Geometry check sheet. Reference: the model listing, model coordinates, mm. Face numbers are marked on the shaded views. Round coordinates to 2 decimals unless told otherwise and drop trailing zeros. Loops run counter-clockwise (first coordinate to the right, second up) from the corner with the lowest first, then second, coordinate; pieces in that order, holes last.
```python
from build123d import *

# Parameters (mm, degrees)
SKETCH1_R           = 38.5
SKETCH1_R_2         = 36.5
BOSS_EXTRUDE1_DEPTH = 257
SKETCH3_W           = 21
SKETCH3_H           = 31
CUT_EXTRUDE1_DEPTH  = 50
SKETCH8_W           = 16.314187307
SKETCH8_H           = 32.341181037
CUT_EXTRUDE4_DEPTH  = 40


with BuildPart() as part:
    # Sketch1 → Boss-Extrude1 (new body)
    with BuildSketch(Plane(origin=(0, 0, 0), x_dir=(1, 0, 0), z_dir=(0, 1, 0))):
        with Locations(Location((0, 0, 0), (0, 0, 270))):
            Circle(SKETCH1_R)
        with Locations(Location((0, 0, 0), (0, 0, 270))):
            Circle(SKETCH1_R_2, mode=Mode.SUBTRACT)
    extrude(amount=BOSS_EXTRUDE1_DEPTH)

    # Sketch3 → Cut-Extrude1 (cut)
    with BuildSketch(Plane(origin=(0, 0, 0), x_dir=(0, 0, -1), z_dir=(1, 0, 0))):
        with Locations((-19.608340935, 67.295682387)):
            Rectangle(SKETCH3_W, SKETCH3_H)
    extrude(amount=-CUT_EXTRUDE1_DEPTH, mode=Mode.SUBTRACT)

    # Sketch8 → Cut-Extrude4 (cut)
    with BuildSketch(Plane.XY):
        with Locations((22.858818879, 14.180131948)):
            Rectangle(SKETCH8_W, SKETCH8_H)
    extrude(amount=CUT_EXTRUDE4_DEPTH, mode=Mode.SUBTRACT)


solid = part.part
```
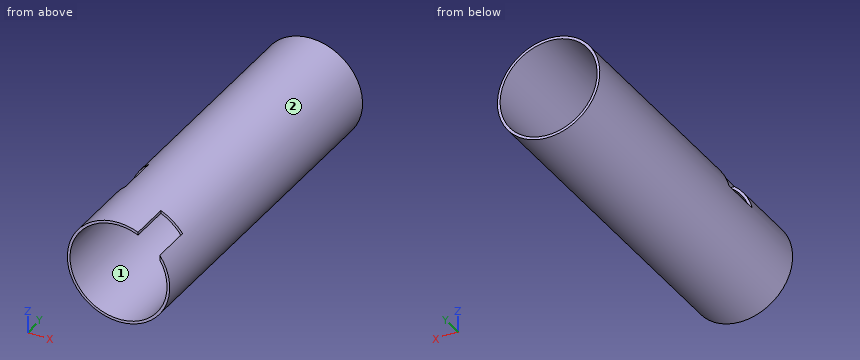
1) Sectioned sample at C-C, the plane x = -31.5. Record the cut outline in (y, z).
Report:
outline: (0, -22.14) - (257, -22.14) - (257, -18.44) - (0, -18.44) - close; (0, 18.44) - (51.8, 18.44) - (51.8, 22.14) - (0, 22.14) - close; (82.8, 18.44) - (257, 18.44) - (257, 22.14) - (82.8, 22.14) - close
2) Sectioned sample at D-D, the plane y = 91.5. Record the cut outline in (x, z).
Report:
outline: circle Ø77 at (0, 0); hole circle Ø73 at (0, 0)
3) Scan lines: line 1 along Z through (x, y) = (-1.5, 112.5); line 2 along X through (y, z) = (114, 0); line 3 along X through (y, z) = (20, 19). Record each from-to range of solid material in increasing order.
Report:
line 1: z = -38.47 to -36.47, 36.47 to 38.47
line 2: x = -38.5 to -36.5, 36.5 to 38.5
line 3: x = -33.49 to -31.16, 31.16 to 33.49
4) Sectioned sample at A-A, the plane x = 0. Record the cut outline in (y, z), then the cut area to 3 significant figures.
Report:
outline: (0, -38.5) - (257, -38.5) - (257, -36.5) - (0, -36.5) - close; (0, 36.5) - (257, 36.5) - (257, 38.5) - (0, 38.5) - close
area: 1,030 mm2
5) Gauge pin test, flat ends, axial feed: pin 1 (6 mm diameter, centred on y = 83, z = 29.5, fed in from -X); pin 2 (12 mm diameter, centred on x = -25, y = 174, fed in from -Z); pin 3 (3 mm diameter, centred on y = 97, z = 13.5, fed in from +X); pin 4 (5 mm diameter, centred on x = -29.5, z = 20.5, fed in from +Y). Record the tip position at first contact, or that the pin passes through.
Report:
pin 1: stops at x = -27.93
pin 2: stops at z = -33.49
pin 3: stops at x = 36.58
pin 4: stops at y = 257
6) Sectioned sample at B-B, the plane z = 0. Record the cut outline in (x, y), then the cut area to 3 significant figures.
Report:
outline: (-38.5, 0) - (-36.5, 0) - (-36.5, 257) - (-38.5, 257) - close; (36.5, 0) - (38.5, 0) - (38.5, 257) - (36.5, 257) - close
area: 1,030 mm2
7) Mould release check, pull along Z, two halves, no side actions. Record for the marked faces 1 and 2: +Z half, -Z half, draft (parallel to the pull), parting line (faces both ways), or undercut.
Report:
face 1: undercut
face 2: parting line
